Could you check a few things on this model? Use its own coordinates, in mm. Face numbers are marked on the shaded views. A direction names the side the tool comes from. Give positions to 0.01 mm unless a question says otherwise; leave off trailing zeros. Order: outer loops, then holes, each group sorted by start corner. A loop starts at its lowest first (then second) coordinate and runs counter-clockwise, first axis right, second up.
from build123d import *

# Parameters (mm, degrees)
CYLINDER_R             = 5
CYLINDER_DEPTH         = 4.5
FILLET_R               = 1
CYLINDER001_R          = 6
CYLINDER001_DEPTH      = 1
BOX001_W               = 30.48
BOX001_H               = 4
BOX001_DEPTH           = 0.5
BOX001_PLACEMENT_ANGLE = 90
BOX_W                  = 30.48
BOX_H                  = 4
BOX_DEPTH              = 0.5
POCKET_DEPTH           = 0.5
ARRAY_COUNT            = 4


with BuildPart() as button_body_fillet:
    # Cylinder → Cylinder (new body)
    with BuildSketch(Plane.XY.offset(8)):
        Circle(CYLINDER_R)
    extrude(amount=CYLINDER_DEPTH)

    # Fillet
    fillet_edges = [button_body_fillet.edges().sort_by_distance(p)[0] for p in [
        (-5, 0, 12.5),
    ]]
    fillet(fillet_edges, radius=FILLET_R)


with BuildPart() as button_fusion:
    # Cylinder001 → Cylinder001 (new body)
    with BuildSketch(Plane.XY.offset(8)):
        Circle(CYLINDER001_R)
    extrude(amount=CYLINDER001_DEPTH)

    # Fusion: union button-body-fillet
    add(button_body_fillet.part)


with BuildPart() as buttons_forward_backward_union_cube:
    # Box001 → Box001 (new body)
    with BuildSketch(Plane.XY):
        with Locations((15.24, 2)):
            Rectangle(BOX001_W, BOX001_H)
    extrude(amount=BOX001_DEPTH)


with BuildPart() as buttons_forward_backward_union_cube_1:
    # Box001 placement: moved
    add(buttons_forward_backward_union_cube.part.moved(Location((2, -15.24, 8))).rotate(Axis((2, -15.24, 8), (0, 0, 1)), BOX001_PLACEMENT_ANGLE))


with BuildPart() as buttons_left_right_union_cube:
    # Box → Box (new body)
    with BuildSketch(Plane(origin=(-15.24, -2, 8), x_dir=(1, 0, 0), z_dir=(0, 0, 1))):
        with Locations((15.24, 2)):
            Rectangle(BOX_W, BOX_H)
    extrude(amount=BOX_DEPTH)


with BuildPart() as buttons_fusion:
    # Clone base: copy of button-fusion
    add(button_fusion.part)


with BuildPart() as buttons_fusion_1:
    # Clone placement: moved
    add(buttons_fusion.part.moved(Location((15.24, 0, 0))))

    # Sketch → Pocket (cut)
    with BuildSketch(Plane(origin=(15.24, 0, 12.5), x_dir=(1, 0, 0), z_dir=(0, 0, 1))):
        Polygon((-1.625, 2.814583), (-1.625, -2.814583), (3.25, 0), align=None)
    extrude(amount=-POCKET_DEPTH, mode=Mode.SUBTRACT)

    # Array: buttons-fusion ×4 about axis
    array_axis = Axis((0, 0, 0), (0, 0, 1))


with BuildPart() as buttons_fusion_2:
    add(buttons_fusion_1.part)
    for i in range(1, ARRAY_COUNT):
        add(buttons_fusion_1.part.rotate(array_axis, i * 360 / ARRAY_COUNT))

    # Fusion001: union button-fusion, buttons-forward-backward-union-cube, buttons-left-right-union-cube
    add(button_fusion.part)
    add(buttons_forward_backward_union_cube_1.part)
    add(buttons_left_right_union_cube.part)


solid = buttons_fusion_2.part
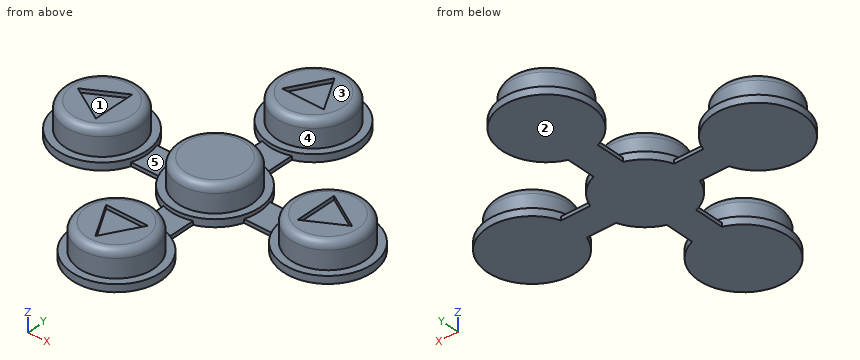
Item 1: Imagine slicing it at B-B on x = -8. List the corners of the cut face in (y, z) for me.
Findings:
outline: (-2, 8) - (2, 8) - (2, 8.5) - (-2, 8.5) - close
Item 2: Imagine slicing it at C-C on y = 15.24. List the corners of the cut face in (x, z) for me.
Findings:
outline: (-6, 8) - (6, 8) - (6, 9) - (5, 9) - (5, 11.5) arc R1 ccw to (4, 12.5) - (1.88, 12.5) - (1.88, 12) - (-1.88, 12) - (-1.88, 12.5) - (-4, 12.5) arc R1 ccw to (-5, 11.5) - (-5, 9) - (-6, 9) - close
Item 3: For the marked faces 1 and 2, which set-ups out of +Z, -Z, +X, -X, +Y, -Y let a thin tool reach every point of the face, with its end or its side?
Findings:
face 1: +Z
face 2: -Z, +X, -X, +Y, -Y
Item 4: For pin 1 (2.5 mm diameter, centred on x = 0.5, y = -15, fed in from +Z); pin 2 (0.6 mm diameter, centred on y = 7.5, z = 8.5, fed in from +X); pin 3 (1.5 mm diameter, centred on y = 15, z = 11, fed in from -X), each with a flat end and sliding along its axis, tell me the tip position at first contact or that it passes through.
Findings:
pin 1: stops at z = 12
pin 2: stops at x = 2
pin 3: stops at x = -5
Item 5: Imagine slicing it at A-A on z = 10.2. List the corners of the cut face in (x, y) for me.
Findings:
outline: circle Ø10 at (-15.24, 0); circle Ø10 at (0, -15.24); circle Ø10 at (0, 0); circle Ø10 at (0, 15.24); circle Ø10 at (15.24, 0)
Item 6: We'd pull the mould along X, two halves only. Please class the marked faces 3, 4 and 5: +X half, -X half, draft (parallel to the pull), parting line (faces both ways), or undercut.
Findings:
face 3: draft
face 4: parting line
face 5: undercut
Item 7: Please list where these lines run through material, in increasing order: line 1 along X through (y, z) = (-1, 10); line 2 along Y through (x, z) = (-4.5, 9.45); line 3 along Y through (x, z) = (4, 12).
Findings:
line 1: x = -20.14 to -10.34, -4.9 to 4.9, 10.34 to 20.14
line 2: y = -17.42 to -13.06, -2.18 to 2.18, 13.06 to 17.42
line 3: y = -18.01 to -12.47, -2.77 to 2.77, 12.47 to 18.01
